The model under review builds one solid part; all positions refer to its coordinate system, in mm. Face numbers are marked on the shaded views. A direction names the side the tool comes from. Give positions to 0.01 mm unless a question says otherwise; leave off trailing zeros. Order: outer loops, then holes, each group sorted by start corner. A loop starts at its lowest first (then second) coordinate and runs counter-clockwise, first axis right, second up. Notation, with made-up numbers: (6.25, 77) - (40.25, 77) arc R12 cw to (40.25, 90) - close; hole circle Ø5 at (50.25, 52). An arc over 180 degrees is marked (long way). Put each result on its own line as item: value.
```python
from build123d import *

# Parameters (mm, degrees)
SKETCH_1_W                = 130
SKETCH_1_H                = 60
EXTRUDE_1_DEPTH           = 12
SKETCH_4_R                = 16.5
EXTRUDE_2_DEPTH           = 6
HOLE_WIZARD_M10_1_D       = 8.5
HOLE_WIZARD_M10_1_DEPTH   = 24.5
HOLE_WIZARD_M10_1_TIP     = 2.553657631
HOLE_WIZARD_1_D           = 5.5
HOLE_WIZARD_1_DEPTH       = 15
HOLE_WIZARD_1_CBORE_D     = 10
HOLE_WIZARD_1_CBORE_DEPTH = 5.7
HOLE_WIZARD_1_TIP         = 1.652366702
CHAMFER_1_SIZE            = 10
CHAMFER_2_SIZE            = 1
SKETCH_7_R                = 14
CUT_EXTRUDE_1_DEPTH       = 73.587877776
CHAMFER_3_SIZE            = 1
SKETCH_8_R                = 22.5
SKETCH_8_R_2              = 7.5
CUT_EXTRUDE_2_DEPTH       = 5
CHAMFER_4_SIZE            = 1


with BuildPart() as part:
    # 草图1 → 凸台-拉伸1 (new body)
    with BuildSketch(Plane.XY):
        Rectangle(SKETCH_1_W, SKETCH_1_H)
    extrude(amount=EXTRUDE_1_DEPTH)

    # 草图4 → 凸台-拉伸2 (add)
    with BuildSketch(Plane(origin=(0, 0, 0), x_dir=(-1, 0, 0), z_dir=(0, 0, -1))):
        Circle(SKETCH_4_R)
    extrude(amount=EXTRUDE_2_DEPTH)

    # M10 螺纹孔1
    with Locations(Plane(origin=(0, 0, -6), x_dir=(-1, 0, 0), z_dir=(0, 0, -1))):
        with Locations((0, 0)):
            Hole(HOLE_WIZARD_M10_1_D / 2, depth=HOLE_WIZARD_M10_1_DEPTH)
            with Locations((0, 0, -(HOLE_WIZARD_M10_1_DEPTH + HOLE_WIZARD_M10_1_TIP / 2))):  # 118° drill point
                Cone(0, HOLE_WIZARD_M10_1_D / 2, HOLE_WIZARD_M10_1_TIP, mode=Mode.SUBTRACT)

    # 打孔尺寸(%根据)内六角圆柱头螺钉的类型1
    with Locations(Plane(origin=(0, 0, 0), x_dir=(-1, 0, 0), z_dir=(0, 0, -1))):
        with Locations((-55, 15), (-55, -15), (-25, 15), (-25, -15), (55, -15), (25, 15), (25, -15), (55, 15)):
            CounterBoreHole(HOLE_WIZARD_1_D / 2, HOLE_WIZARD_1_CBORE_D / 2, HOLE_WIZARD_1_CBORE_DEPTH, depth=HOLE_WIZARD_1_DEPTH)
            with Locations((0, 0, -(HOLE_WIZARD_1_DEPTH + HOLE_WIZARD_1_TIP / 2))):  # 118° drill point
                Cone(0, HOLE_WIZARD_1_D / 2, HOLE_WIZARD_1_TIP, mode=Mode.SUBTRACT)

    # 倒角1
    chamfer_1_edges = [part.edges().sort_by_distance(p)[0] for p in [
        (65, -30, 6),
        (-65, -30, 6),
        (-65, 30, 6),
        (65, 30, 6),
    ]]
    chamfer(chamfer_1_edges, length=CHAMFER_1_SIZE)

    # 倒角2
    chamfer_2_edges = [part.edges().sort_by_distance(p)[0] for p in [
        (0, -30, 0),
        (0, -30, 12),
        (65, 0, 0),
        (-65, 0, 0),
        (0, 30, 0),
        (60, 25, 0),
        (60, -25, 0),
        (-60, 25, 0),
        (-60, -25, 0),
        (-65, 0, 12),
        (65, 0, 12),
        (0, 30, 12),
        (60, 25, 12),
        (60, -25, 12),
        (-60, 25, 12),
        (-60, -25, 12),
    ]]
    chamfer(chamfer_2_edges, length=CHAMFER_2_SIZE)

    # 草图7 → 切除-拉伸1 (cut, through all)
    with BuildSketch(Plane(origin=(0, 0, 0), x_dir=(-1, 0, 0), z_dir=(0, 0, -1))):
        with Locations((-40, 0)):
            Circle(SKETCH_7_R)
        with Locations((40, 0)):
            Circle(SKETCH_7_R)
    extrude(amount=-CUT_EXTRUDE_1_DEPTH, mode=Mode.SUBTRACT)

    # 倒角3
    chamfer_3_edges = [part.edges().sort_by_distance(p)[0] for p in [
        (54, 0, 12),
        (54, 0, 0),
        (-26, 0, 12),
        (-26, 0, 0),
    ]]
    chamfer(chamfer_3_edges, length=CHAMFER_3_SIZE)

    # 草图8 → 切除-拉伸2 (cut)
    with BuildSketch(Plane.XY.offset(12)):
        Circle(SKETCH_8_R)
        Circle(SKETCH_8_R_2, mode=Mode.SUBTRACT)
    extrude(amount=-CUT_EXTRUDE_2_DEPTH, mode=Mode.SUBTRACT)

    # 倒角4
    chamfer_4_edges = [part.edges().sort_by_distance(p)[0] for p in [
        (-22.5, 0, 12),
        (-7.5, 0, 12),
    ]]
    chamfer(chamfer_4_edges, length=CHAMFER_4_SIZE)


solid = part.part
```
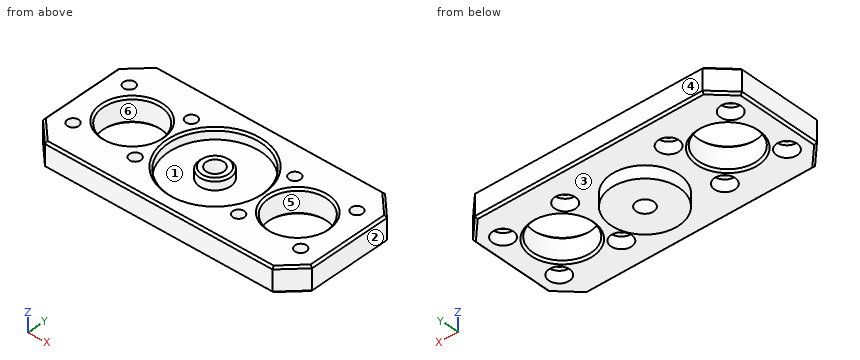
(1) For the marked faces 1 and 2, list the 3-axis set-ups (+Z, -Z, +X, -X, +Y, -Y) from which the entire face can be reached by the end or side of a thin tool; tool diameter is ignored.
The answers:
face 1: +Z
face 2: +Z, -Z, +X, +Y, -Y
(2) Clearance check with flat-ended pins moving along their axes: pin 1 Ø6.5 at (x, y) = (-55, 15) entering from -Z; pin 2 Ø11 at (x, y) = (-25.5, 15.5) entering from -Z; pin 3 Ø8 at (x, y) = (25, 15) entering from +Z. State where each tip first meets the part, or that it passes through.
The answers:
pin 1: z = 5.7
pin 2: z = 0
pin 3: z = 12
(3) Take a section at D-D, the plane z = -1.5. Write out the cut boundary in (x, y), then the cut area to 3 significant figures.
The answers:
outline: circle Ø33 at (0, 0); hole circle Ø8.5 at (0, 0)
area: 799 mm^2
(4) Take a section at A-A, the plane z = 8.75. Count the separate pieces of the cut face and the enclosed holes in it, then the cut area to 3 significant figures.
The answers:
separate pieces: 2
enclosed holes: 12
area: 4,710 mm^2
(5) The part is to be moulded in two halves that separate along Y. For the marked faces 3, 4, 5 and 6, say which applies: pulls with the +Y half, pulls with the -Y half, needs draft (parallel to the pull), parting line crosses it, or undercut.
The answers:
face 3: needs draft
face 4: pulls with the +Y half
face 5: undercut
face 6: undercut
(6) Wall thickness on L1, parallel to Y at x = 25, z = 10; L2, parallel to Y at x = 55, z = 4.55; L3, parallel to X at y = 18, z = 0.75: over which ranges is each line inside the solid? List them lowest first.
The answers:
L1: -30 to -17.75, -12.25 to 12.25, 17.75 to 30
L2: -30 to -20, -10 to 10, 20 to 30
L3: -64.75 to -59, -51 to -29, -21 to 21, 29 to 51, 59 to 64.75
(7) Take a section at B-B, the plane x = 0. Write out the cut boundary in (y, z).
The answers:
outline: (-30, 1) - (-29, 0) - (-16.5, 0) - (-16.5, -6) - (-4.25, -6) - (-4.25, 12) - (-6.5, 12) - (-7.5, 11) - (-7.5, 7) - (-22.5, 7) - (-22.5, 11) - (-23.5, 12) - (-29, 12) - (-30, 11) - close; (4.25, -6) - (16.5, -6) - (16.5, 0) - (29, 0) - (30, 1) - (30, 11) - (29, 12) - (23.5, 12) - (22.5, 11) - (22.5, 7) - (7.5, 7) - (7.5, 11) - (6.5, 12) - (4.25, 12) - close
